The figure shows three views and two pictorial views of one solid part (mm, origin at its lowest corner). Answer the questions. Coordinates: 2 decimals unless noted, no trailing zeros. Write each loop counter-clockwise with the first axis right and the second up, starting at its lowest first coordinate (ties: lowest second). Pieces come first, ordered by that corner, then holes. Notation, with made-up numbers: M -30.75,-14.5 L 5.25,-14.5 A22 cw 5.25,2.5 Z; hole C 64.25,10.25 d7. An arc over 180 degrees is marked long. Write item = value, one per line.
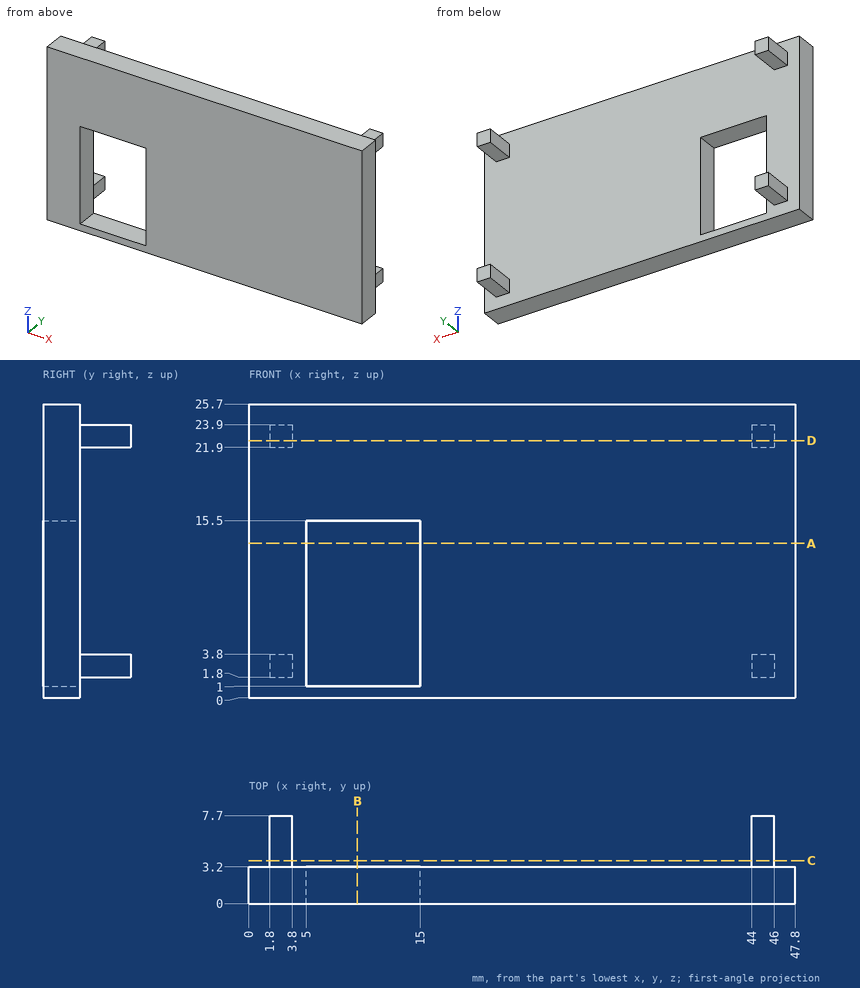
Item 1: Find section A-A (z = 13.5). Determine the outline of the cut face in (x, y).
Worked answers:
outline = M 0,0 L 5,0 L 5,3.2 L 0,3.2 Z; M 15,0 L 47.8,0 L 47.8,3.2 L 15,3.2 Z
Item 2: Find section B-B (x = 9.5). Determine the outline of the cut face in (y, z), and give its area (3 significant figures).
Worked answers:
outline = M 0,0 L 3.2,0 L 3.2,1 L 0,1 Z; M 0,15.5 L 3.2,15.5 L 3.2,25.7 L 0,25.7 Z
area = 35.8 mm²
Item 3: Find section D-D (z = 22.5). Determine the outline of the cut face in (x, y), and give its area (3 significant figures).
Worked answers:
outline = M 0,0 L 47.8,0 L 47.8,3.2 L 46,3.2 L 46,7.7 L 44,7.7 L 44,3.2 L 3.8,3.2 L 3.8,7.7 L 1.8,7.7 L 1.8,3.2 L 0,3.2 Z
area = 171 mm²
Item 4: Find section C-C (y = 3.75). Determine the outline of the cut face in (x, z), and give its area (3 significant figures).
Worked answers:
outline = M 1.8,1.8 L 3.8,1.8 L 3.8,3.8 L 1.8,3.8 Z; M 1.8,21.9 L 3.8,21.9 L 3.8,23.9 L 1.8,23.9 Z; M 44,1.8 L 46,1.8 L 46,3.8 L 44,3.8 Z; M 44,21.9 L 46,21.9 L 46,23.9 L 44,23.9 Z
area = 16.0 mm²
Item 5: Flat-ended cylindrical pins translate along their axes: pin 1 (1 mm diameter, centred on x = 23, z = 18, fed in from +Y); pin 2 (1 mm diameter, centred on y = 6, z = 2.5, fed in from +X); pin 3 (1 mm diameter, centred on x = 3, y = 6.5, fed in from -Z). Find the tip coordinate at first contact, or state that the pin passes through.
Worked answers:
pin_1 = 3.2
pin_2 = 46
pin_3 = 1.8
Item 6: Consider line 1 along X through (y, z) = (2.25, 9.75); line 2 along Y through (x, z) = (41, 21.5). Determine where each line is inside the solid, lowest interval first. Write a range as from..to.
Worked answers:
line_1 = 0..5, 15..47.8
line_2 = 0..3.2
